Part model, mm, in its own coordinate system. A direction names the side the tool comes from. Round coordinates to 2 decimals unless told otherwise and drop trailing zeros. Write each loop counter-clockwise with the first axis right and the second up, starting at its lowest first coordinate (ties: lowest second). Pieces come first, ordered by that corner, then holes.
```python
from build123d import *

# Parameters (mm, degrees)
SKETCH2_W           = 60
SKETCH2_H           = 45
BOSS_EXTRUDE1_DEPTH = 13
BOSS_EXTRUDE2_DEPTH = 45
SKETCH11_W          = 60
SKETCH11_H          = 10
SKETCH11_H_2        = 6.608108108
CUT_EXTRUDE2_DEPTH  = 21
BOSS_EXTRUDE3_REACH = 42
SKETCH12_W          = 20
SKETCH12_H          = 35
DRAFT1_ANGLE        = -15
CUT_EXTRUDE3_DEPTH  = 46


with BuildPart() as part:
    # Sketch2 → Boss-Extrude1 (new body)
    with BuildSketch(Plane(origin=(0, 0, 0), x_dir=(1, 0, 0), z_dir=(0, 1, 0))):
        Rectangle(SKETCH2_W, SKETCH2_H)
    extrude(amount=BOSS_EXTRUDE1_DEPTH)

    # Sketch3 → Boss-Extrude2 (add)
    with BuildSketch(Plane.XY.offset(22.5)):
        Polygon((0, 30.320508076), (30, 13), (-30, 13), align=None)
    extrude(amount=-BOSS_EXTRUDE2_DEPTH)

    # Sketch11 → Cut-Extrude2 (cut)
    with BuildSketch(Plane(origin=(0, 38, 0), x_dir=(-1, 0, 0), z_dir=(0, -1, 0))):
        with Locations((0, 17.5)):
            Rectangle(SKETCH11_W, SKETCH11_H)
        with Locations((0, -19.195945946)):
            Rectangle(SKETCH11_W, SKETCH11_H_2)
    extrude(amount=CUT_EXTRUDE2_DEPTH, mode=Mode.SUBTRACT)

    # Sketch12 → Boss-Extrude3 (add, up to next)
    with BuildSketch(Plane(origin=(0, 40, 0), x_dir=(-1, 0, 0), z_dir=(0, -1, 0)), mode=Mode.PRIVATE) as boss_extrude3_sk1:
        with Locations((0, -5)):
            Rectangle(SKETCH12_W, SKETCH12_H)
    boss_extrude3_tool1 = extrude(boss_extrude3_sk1.sketch, amount=BOSS_EXTRUDE3_REACH, mode=Mode.PRIVATE) - part.part
    add(boss_extrude3_tool1.solids().sort_by_distance((0, 40, 5))[0])

    # Draft1
    draft1_faces = [part.faces().sort_by_distance(p)[0] for p in [
        (0, 40, 5),
    ]]
    draft(draft1_faces, Plane(origin=(30, 13, 22.5), x_dir=(1, 0, 0), z_dir=(0, 0, 1)), DRAFT1_ANGLE)

    # Sketch16 → Cut-Extrude3 (cut, through all)
    with BuildSketch(Plane(origin=(0, 0, -22.5), x_dir=(-1, 0, 0), z_dir=(0, 0, -1))):
        Polygon((-12.886751346, 5), (-10, 0), (10, 0), (12.886751346, 5), align=None)
    extrude(amount=-CUT_EXTRUDE3_DEPTH, mode=Mode.SUBTRACT)


solid = part.part
```
Q1. Cut at A-A on y = 3. Write the cut outline in (x, z), plus the area to 3 significant figures.
Values follow:
outline: (-30, -22.5) - (-11.73, -22.5) - (-11.73, 22.5) - (-30, 22.5) - close; (11.73, -22.5) - (30, -22.5) - (30, 22.5) - (11.73, 22.5) - close
area: 1,640 mm2
Q2. Which spindle directions (+Z, -Z, +X, -X, +Y, -Y) get a long thin tool onto all of the face, cutting with end or side? Do faces 1 (the flat face through (-11.423, 2.465, -0.315)), 2 (the flat face through (0, 22, -12.5)), 3 (the flat face through (10, 29, 9)), 4 (the flat face through (-16, 17, 19)). Say none if no direction does.
Values follow:
face 1: +Z, -Z
face 2: -Z, +X, -X, +Y
face 3: +Z, +X, +Y
face 4: +Z, -X, +Y
Q3. Mould opens along X. For faces 5 (the flat face through (0, 16, 22.5)), 6 (the flat face through (11.46, 2.53, -0.32)), 7 (the flat face through (30, 6, 0)) say: +X half, -X half, draft (parallel to the pull), parting line (faces both ways), or undercut.
Values follow:
face 5: draft
face 6: undercut
face 7: +X half
Q4. Cut at C-C on x = -5.5. Write the cut outline in (y, z).
Values follow:
outline: (5, -22.5) - (17, -22.5) - (17, -12.5) - (30.62, -12.5) - (40, 22.5) - (5, 22.5) - close
Q5. Wall check: L1, parallel to Y at x = 13, z = 16; L2, parallel to X at y = 2.5, z = -15.5; L3, parallel to X at y = 29.5, z = 4.5. Give the ranges that are in metal, low to high.
Values follow:
L1: y = 0 to 17
L2: x = -30 to -11.44, 11.44 to 30
L3: x = -10 to 10
Q6. Cut at B-B on z = -19. Write the cut outline in (x, y), plus the area to 3 significant figures.
Values follow:
outline: (-30, 0) - (-10, 0) - (-12.89, 5) - (12.89, 5) - (10, 0) - (30, 0) - (30, 13) - (23.07, 17) - (-23.07, 17) - (-30, 13) - close
area: 878 mm2
Q7. Cut at D-D on y = 23.5. Write the cut outline in (x, z), plus the area to 3 significant figures.
Values follow:
outline: (-11.81, -12.5) - (11.81, -12.5) - (11.81, 15.89) - (10, 15.89) - (10, 22.5) - (-10, 22.5) - (-10, 15.89) - (-11.81, 15.89) - close
area: 803 mm2
Q8. Drop flat-ended pins along their axis: pin 1 (3.5 mm diameter, centred on x = 14, z = 18, fed in from +Y); pin 2 (15 mm diameter, centred on x = 8.5, y = 22, fed in from -Z); pin 3 (8.5 mm diameter, centred on x = -17.5, y = 21.5, fed in from +Z); pin 4 (18.5 mm diameter, centred on y = 33, z = 2, fed in from +X). Give the stop position or say it passes through.
Values follow:
pin 1: stops at y = 17
pin 2: stops at z = -22.5
pin 3: stops at z = 15.89
pin 4: stops at x = 11.38
